Part model, mm, in its own coordinate system. A direction names the side the tool comes from. Round coordinates to 2 decimals unless told otherwise and drop trailing zeros. Loops run counter-clockwise (first coordinate to the right, second up) from the corner with the lowest first, then second, coordinate; pieces in that order, holes last. Notation, with made-up numbers: M 76.25,67.5 L 81.25,67.5 A19 cw 81.25,73.5 Z; hole C -34.75,36 d9. An arc over 180 degrees is marked long. Write each question's results on one line, items separated by ' | '.
from build123d import *

# Parameters (mm, degrees)
BOSS_EXTRUDE1_DEPTH = 35
SKETCH3_R           = 9.5
CUT_EXTRUDE1_DEPTH  = 5
SKETCH4_R           = 5
CUT_EXTRUDE2_DEPTH  = 31
SKETCH5_R           = 2.5
CUT_EXTRUDE3_DEPTH  = 26.656854249


with BuildPart() as part:
    # Sketch2 → Boss-Extrude1 (new body)
    with BuildSketch(Plane.XY):
        Polygon((-5, 0), (5, 0), (10.656854249, 5.656854249), (19, 5.656854249), (19, 15.656854249), (20, 17.656854249), (20, 25.656854249), (-20, 25.656854249), (-20, 17.656854249), (-19, 15.656854249), (-19, 5.656854249), (-10.656854249, 5.656854249), align=None)
    extrude(amount=BOSS_EXTRUDE1_DEPTH)

    # Sketch3 → Cut-Extrude1 (cut)
    with BuildSketch(Plane.XY.offset(35)):
        with Locations((0, 12.828427125)):
            Circle(SKETCH3_R)
    cut_extrude1 = extrude(amount=-CUT_EXTRUDE1_DEPTH, mode=Mode.SUBTRACT)

    # Sketch4 → Cut-Extrude2 (cut, through all)
    with BuildSketch(Plane.XY.offset(30)):
        with Locations((0, 12.828427125)):
            Circle(SKETCH4_R)
    extrude(amount=-CUT_EXTRUDE2_DEPTH, mode=Mode.SUBTRACT)

    # Mirror1: Cut-Extrude1 across plane
    add(cut_extrude1.mirror(Plane.XY.offset(17.5)), mode=Mode.SUBTRACT)

    # Sketch5 → Cut-Extrude3 (cut, through all)
    with BuildSketch(Plane(origin=(0, 25.656854249, 0), x_dir=(1, 0, 0), z_dir=(0, 1, 0))):
        with Locations((-14, -7)):
            Circle(SKETCH5_R)
        with Locations((14, -7)):
            Circle(SKETCH5_R)
        with Locations((14, -28)):
            Circle(SKETCH5_R)
        with Locations((-14, -28)):
            Circle(SKETCH5_R)
    extrude(amount=-CUT_EXTRUDE3_DEPTH, mode=Mode.SUBTRACT)


solid = part.part
Item 1: Band-saw the part on A-A on x = 14. Give the cut face in (y, z).
Filled sheet:
outline: M 5.66,0 L 25.66,0 L 25.66,4.5 L 5.66,4.5 Z; M 5.66,9.5 L 25.66,9.5 L 25.66,25.5 L 5.66,25.5 Z; M 5.66,30.5 L 25.66,30.5 L 25.66,35 L 5.66,35 Z
Item 2: Band-saw the part on D-D on y = 14. Give the cut face in (x, z).
Filled sheet:
outline: M -19,0 L -9.43,0 L -9.43,5 L -4.86,5 L -4.86,30 L -9.43,30 L -9.43,35 L -19,35 Z; M 4.86,5 L 9.43,5 L 9.43,0 L 19,0 L 19,35 L 9.43,35 L 9.43,30 L 4.86,30 Z; hole C -14,7 d5; hole C -14,28 d5; hole C 14,7 d5; hole C 14,28 d5
Item 3: Which spindle directions (+Z, -Z, +X, -X, +Y, -Y) get a long thin tool onto all of the face, cutting with end or side? Do faces 1 (the flat face through (0, 0, 17)), 2 (the flat face through (19, 11, 17)), 3 (the flat face through (4, 9, 30)), 4 (the flat face through (4, 9, 5)). Say none if no direction does.
Filled sheet:
face 1: +Z, -Z, +X, -X, -Y | face 2: +Z, -Z, +X, -Y | face 3: +Z | face 4: -Z
Item 4: Band-saw the part on C-C on x = 0. Give the cut face in (y, z), and give its area (3 significant figures).
Filled sheet:
outline: M 0,0 L 3.33,0 L 3.33,5 L 7.83,5 L 7.83,30 L 3.33,30 L 3.33,35 L 0,35 Z; M 17.83,5 L 22.33,5 L 22.33,0 L 25.66,0 L 25.66,35 L 22.33,35 L 22.33,30 L 17.83,30 Z | area: 458 mm^2
Item 5: Drop flat-ended pins along their axis: P1, Ø3, axis at y = 9.5, z = 9.5, coming from the -X side; P2, Ø6, axis at x = -14, z = 7, coming from the -Y side; P3, Ø5, axis at x = 10.5, z = 24, coming from the -Y side; P4, Ø3, axis at x = 14, z = 7, coming from the -Y side. Give the stop position or say it passes through.
Filled sheet:
P1: x = -19 | P2: y = 5.66 | P3: y = 3 | P4: through
Item 6: Band-saw the part on B-B on z = 7. Give the cut face in (x, y).
Filled sheet:
outline: M -20,17.66 L -19,15.66 L -19,5.66 L -16.5,5.66 L -16.5,25.66 L -20,25.66 Z; M -11.5,5.66 L -10.66,5.66 L -5,0 L 5,0 L 10.66,5.66 L 11.5,5.66 L 11.5,25.66 L -11.5,25.66 Z; M 16.5,5.66 L 19,5.66 L 19,15.66 L 20,17.66 L 20,25.66 L 16.5,25.66 Z; hole C 0,12.83 d10
Item 7: Wall check: L1, parallel to Z at x = 14, y = 14; L2, parallel to X at y = 21.5, z = 7; L3, parallel to X at y = 12.5, z = 7. Give the ranges that are in metal, low to high.
Filled sheet:
L1: 0 to 4.5, 9.5 to 25.5, 30.5 to 35 | L2: -20 to -16.5, -11.5 to 11.5, 16.5 to 20 | L3: -19 to -16.5, -11.5 to -4.99, 4.99 to 11.5, 16.5 to 19
Item 8: Two-plate mould, pull along X, no slides. Class faces 5 (the flat face through (19.49, 16.64, 17.26)), 6 (the cylindrical face through (-2.059, 3.554, 2.465)), 7 (the flat face through (-5, 22, 0)), 8 (the flat face through (-19, 11, 17)): +X half, -X half, draft (parallel to the pull), parting line (faces both ways), or undercut.
Filled sheet:
face 5: +X half | face 6: undercut | face 7: draft | face 8: -X half
